from build123d import *

# Parameters (mm, degrees)
F1_DEPTH = 25.4
F2_DEPTH = 6.35
F3_DEPTH = 6.35


with BuildPart() as f1:
    # F0 (on Front) → F1 (new body)
    with BuildSketch(Plane.XZ):
        with BuildLine():
            ThreePointArc((0, 9.525), (-4.7625, 4.7625), (0, 0))
            Line((0, 0), (50.8, 0))
            ThreePointArc((50.8, 0), (55.574371, 5.123585), (50.127052, 9.525))
            Line((50.127052, 9.525), (0, 9.525))
        make_face()
    extrude(amount=F1_DEPTH)

    # F0 (on Front) → F2 (cut)
    with BuildSketch(Plane.XZ):
        with BuildLine():
            ThreePointArc((0, 15.875), (-11.1125, 4.7625), (0, -6.35))
            Line((0, -6.35), (50.8, -6.35))
            ThreePointArc((50.8, -6.35), (61.92438, 5.300794), (49.772055, 15.875))
            Line((49.772055, 15.875), (0, 15.875))
        make_face()
        with BuildLine():
            Line((50.8, 0), (0, 0))
            ThreePointArc((0, 0), (-4.7625, 4.7625), (0, 9.525))
            Line((0, 9.525), (50.127052, 9.525))
            ThreePointArc((50.127052, 9.525), (55.574371, 5.123585), (50.8, 0))
        make_face(mode=Mode.SUBTRACT)
        with BuildLine():
            ThreePointArc((0, 9.525), (-4.7625, 4.7625), (0, 0))
            Line((0, 0), (50.8, 0))
            ThreePointArc((50.8, 0), (55.574371, 5.123585), (50.127052, 9.525))
            Line((50.127052, 9.525), (0, 9.525))
        make_face()
    extrude(amount=-F2_DEPTH, mode=Mode.SUBTRACT)

    # F0 (on Front) → F3 (join)
    with BuildSketch(Plane.XZ):
        with BuildLine():
            ThreePointArc((0, 15.875), (-11.1125, 4.7625), (0, -6.35))
            Line((0, -6.35), (50.8, -6.35))
            ThreePointArc((50.8, -6.35), (61.92438, 5.300794), (49.772055, 15.875))
            Line((49.772055, 15.875), (0, 15.875))
        make_face()
        with BuildLine():
            Line((50.8, 0), (0, 0))
            ThreePointArc((0, 0), (-4.7625, 4.7625), (0, 9.525))
            Line((0, 9.525), (50.127052, 9.525))
            ThreePointArc((50.127052, 9.525), (55.574371, 5.123585), (50.8, 0))
        make_face(mode=Mode.SUBTRACT)
        with BuildLine():
            ThreePointArc((0, 9.525), (-4.7625, 4.7625), (0, 0))
            Line((0, 0), (50.8, 0))
            ThreePointArc((50.8, 0), (55.574371, 5.123585), (50.127052, 9.525))
            Line((50.127052, 9.525), (0, 9.525))
        make_face()
    extrude(amount=-F3_DEPTH)


solid = f1.part
Could you check a few things on this model? Use its own coordinates, in mm. A direction names the side the tool comes from. Coordinates: 2 decimals unless noted, no trailing zeros. Loops run counter-clockwise (first coordinate to the right, second up) from the corner with the lowest first, then second, coordinate; pieces in that order, holes last.
1. Imagine slicing it at B-B (z = 5.25). Please give me the cut outline in (x, y), and give its area (3 significant figures).
2. For faces 1 (the face through (25, 6.35, 5)), 2 (the face through (25, -13, 0)), 3 (the face through (-4.76, -12.52, 4.87)), 4 (the face through (-11.11, 3.13, 5.01)), which set-ups out of +Z, -Z, +X, -X, +Y, -Y let a thin tool reach every point of the face, with its end or its side?
3. I need wall thicknesses on L1, parallel to Z at x = 43.5, y = -10 (3 decimals); L2, parallel to Y at x = 53, z = 0.5; L3, parallel to Z at x = 49.5, y = 3.5 (3 decimals). Which ranges of each line are inside material? Lowest first, please.
4. Imagine slicing it at A-A (x = 41.5). Please give me the cut outline in (y, z) (3 decimals), and give its area (3 significant figures).
5. Imagine slicing it at D-D (y = -8.5). Please give me the cut outline in (x, z) (1 decimal).
6. For P1, Ø12, axis at x = 16, y = -6.5, coming from the -Z side; P2, Ø7.5, axis at x = 26.5, y = -18, coming from the +Z side (3 decimals); P3, Ø7, axis at x = 24.5, y = 4, coming from the +Z side (3 decimals), each with a flat end and sliding along its axis, tell me the tip position at first contact or that it passes through.
Computed values:
1. outline: (-11.1, 0) - (-4.74, 0) - (-4.74, -25.4) - (55.56, -25.4) - (55.56, 0) - (61.93, 0) - (61.93, 6.35) - (-11.1, 6.35) - close
1. area: 2,000 mm2
2. face 1: +Z, -Z, +X, -X, +Y
2. face 2: -Z, +X, -X, -Y
2. face 3: -X, -Y
2. face 4: -X, +Y, -Y
3. L1: z = 0 to 9.525
3. L2: y = 0 to 6.35
3. L3: z = -6.35 to 15.875
4. outline: (-25.4, 0) - (0, 0) - (0, -6.35) - (6.35, -6.35) - (6.35, 15.875) - (0, 15.875) - (0, 9.525) - (-25.4, 9.525) - close
4. area: 383 mm2
5. outline: (0, 0) - (50.8, 0) arc R4.8 ccw (long way) to (50.1, 9.5) - (0, 9.5) arc R4.8 ccw to start
6. P1: stops at z = 0
6. P2: stops at z = 9.525
6. P3: stops at z = 15.875
